Part model, mm, in its own coordinate system. Coordinates: 2 decimals unless noted, no trailing zeros. Use one line per item in the form item = value. Start each with the question number.
(1) Band-saw the part on A-A on x = -48. Count the separate pieces of the cut face and the enclosed holes in it, then the cut area to 3 significant figures.
(2) Drill centre lines: L1, parallel to Z at x = -19.5, y = 2.5; L2, parallel to X at y = 0.75, z = -73. Where is each one in solid material? Low to high. Write a range as [from, to].
(3) Pin check, flat tips, straight feed: P1, Ø4.5, axis at x = 64, z = 0, coming from the -Y side; P2, Ø3, axis at x = -14.5, z = 52, coming from the -Y side. Stop position of each tip, or through.
```python
from build123d import *

# Parameters (mm, degrees)
SKETCH2_W            = 149.225
SKETCH2_H            = 177.8
BOSS_EXTRUDE1_DEPTH  = 6.35
FILLET1_R            = 6.35
SKETCH3_R            = 2.4
CUT_EXTRUDE2_DEPTH   = 7.35
LPATTERN2_COUNT      = 9
LPATTERN2_PITCH      = 16
LPATTERN2_COUNT_DIR2 = 11
LPATTERN2_PITCH_DIR2 = 16
SKETCH4_R            = 1.6
MOUNTING_HOLES_DEPTH = 7.35
SKETCH5_W            = 19.6
SKETCH5_H            = 13
SWITCH_CUTOUT_DEPTH  = 7.35


with BuildPart() as part:
    # Sketch2 → Boss-Extrude1 (new body)
    with BuildSketch(Plane(origin=(0, 0, 0), x_dir=(1, 0, 0), z_dir=(0, 1, 0))):
        Rectangle(SKETCH2_W, SKETCH2_H)
    extrude(amount=BOSS_EXTRUDE1_DEPTH)

    # Fillet1
    fillet1_edges = [part.edges().sort_by_distance(p)[0] for p in [
        (74.6125, 3.175, 88.9),
        (-74.6125, 3.175, 88.9),
        (-74.6125, 3.175, -88.9),
        (74.6125, 3.175, -88.9),
    ]]
    fillet(fillet1_edges, radius=FILLET1_R)

    # Sketch3 → Cut-Extrude2 (cut, through all)
    with BuildSketch(Plane(origin=(0, 6.35, 0), x_dir=(1, 0, 0), z_dir=(0, 1, 0))):
        with Locations((-64, 80)):
            Circle(SKETCH3_R)
    cut_extrude2 = extrude(amount=-CUT_EXTRUDE2_DEPTH, mode=Mode.SUBTRACT)

    # LPattern2: Cut-Extrude2 9 × 11, 2 skipped
    with Locations(*[(i * LPATTERN2_PITCH, 0, j * LPATTERN2_PITCH_DIR2) for i in range(LPATTERN2_COUNT) for j in range(LPATTERN2_COUNT_DIR2) if (i, j) not in ((0, 0), (7, 0), (8, 0))]):
        add(cut_extrude2, mode=Mode.SUBTRACT)

    # Sketch4 → MOUNTING_HOLES (cut, through all)
    with BuildSketch(Plane(origin=(0, 6.35, 0), x_dir=(1, 0, 0), z_dir=(0, 1, 0))):
        with Locations((-69.08, 67.9)):
            Circle(SKETCH4_R)
        with Locations((-20.82, 66.376)):
            Circle(SKETCH4_R)
        with Locations((-20.82, -8.554)):
            Circle(SKETCH4_R)
        with Locations((-69.08, -14.65)):
            Circle(SKETCH4_R)
        with Locations((-64, 15.83)):
            Circle(SKETCH4_R)
        with Locations((-36.314, 15.83)):
            Circle(SKETCH4_R)
    extrude(amount=-MOUNTING_HOLES_DEPTH, mode=Mode.SUBTRACT)

    # Sketch5 → SWITCH_CUTOUT (cut, through all)
    with BuildSketch(Plane(origin=(0, 6.35, 0), x_dir=(1, 0, 0), z_dir=(0, 1, 0))):
        with Locations((56.8125, 77.4)):
            Rectangle(SKETCH5_W, SKETCH5_H)
    extrude(amount=-SWITCH_CUTOUT_DEPTH, mode=Mode.SUBTRACT)


solid = part.part
```
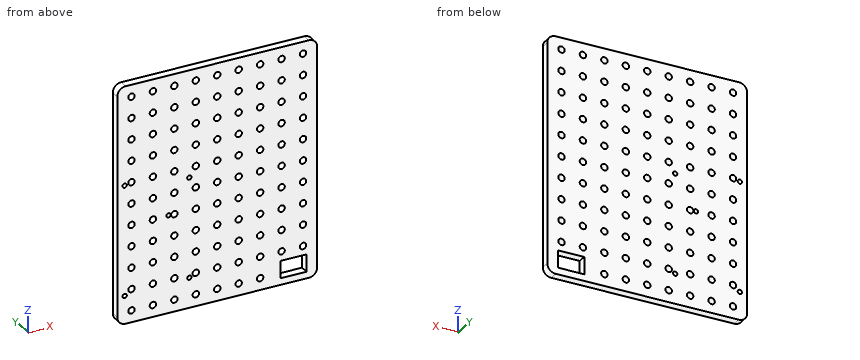
A:
q1.separate_pieces = 12
q1.enclosed_holes = 0
q1.area = 794 mm²
q2.L1 = [-88.9, -67.28], [-65.47, 7.65], [9.46, 88.9]
q2.L2 = [-74.61, 47.01], [66.61, 74.61]
q3.P1 = through
q3.P2 = 0
